Input: part model. Units: mm. Frame: model coordinates. Face numbers are marked on the shaded views. A direction names the side the tool comes from. Coordinates: 2 decimals unless noted, no trailing zeros. Write each loop counter-clockwise with the first axis right and the second up, starting at its lowest first coordinate (ties: lowest second). Pieces come first, ordered by that corner, then holes.
1) Draft query along Z for the marked faces 1, 2 and 3. Return one class per face: pulls with the +Z half, pulls with the -Z half, needs draft (parallel to the pull), parting line crosses it, or undercut.
2) Section query B-B (y = 0). Output: boundary loops of the cut face in (x, z), then the cut area to 3 significant figures.
3) Set-up query: the marked faces 4 and 5. Return all of +Z, -Z, +X, -X, +Y, -Y with unobstructed straight access to the full face (end or side cutting, diameter ignored); none if empty.
4) Pin query (flat end, axial travel): pin 1 Ø1 at (y, z) = (-18, 0.5) entering from +X; pin 2 Ø10 at (x, z) = (4.5, 4.5) entering from +Y; pin 3 Ø7 at (x, y) = (0, 0) entering from +Z; pin 4 Ø2 at (x, z) = (-9, -4) entering from +Y. Return the tip coordinate at first contact, or that it passes through.
5) Section query A-A (z = 0). Output: boundary loops of the cut face in (x, y).
6) Section query D-D (x = 0). Output: boundary loops of the cut face in (y, z), then the cut area to 3 significant figures.
7) Section query C-C (z = -5.75). Output: boundary loops of the cut face in (x, y), then the cut area to 3 significant figures.
8) Line query: L1, parallel to X at y = -54, z = 0; L2, parallel to Y at x = 0, z = 0.55; L3, parallel to Z at x = 8.5, y = -26.5. Output: solid intervals per line, ascending.
from build123d import *

# Parameters (mm, degrees)
SKETCH4_W           = 18
SKETCH4_H           = 18
BOSS_EXTRUDE2_DEPTH = 9
SKETCH5_R           = 3.15
CUT_EXTRUDE1_DEPTH  = 18
SKETCH6_R           = 6
CUT_EXTRUDE2_DEPTH  = 7.25
CUT_EXTRUDE2_DRAFT  = -2
SKETCH8_R           = 6
CUT_EXTRUDE3_DEPTH  = 7.25
CUT_EXTRUDE3_DRAFT  = -2
CHAMFER1_SIZE       = 5
SKETCH13_W          = 18
SKETCH13_H          = 18
BOSS_EXTRUDE4_DEPTH = 50.25
SKETCH14_W          = 35
SKETCH14_H          = 18.08381725
BOSS_EXTRUDE5_DEPTH = 8
SKETCH15_R          = 3.4
CUT_EXTRUDE4_DEPTH  = 8
SKETCH16_R          = 3.4
CUT_EXTRUDE5_DEPTH  = 8


with BuildPart() as part:
    # Sketch4 → Boss-Extrude2 (new, symmetric)
    with BuildSketch(Plane(origin=(0, 0, 0), x_dir=(1, 0, 0), z_dir=(0, 1, 0))):
        Rectangle(SKETCH4_W, SKETCH4_H)
    extrude(amount=BOSS_EXTRUDE2_DEPTH, both=True)

    # Sketch5 → Cut-Extrude1 (cut)
    with BuildSketch(Plane.XY.offset(9)):
        Circle(SKETCH5_R)
    extrude(amount=-CUT_EXTRUDE1_DEPTH, mode=Mode.SUBTRACT)


with BuildPart() as cut_extrude2_tool:
    # Sketch6 → Cut-Extrude2 (with draft: the straight prism first)
    with BuildSketch(Plane.XY.offset(9)):
        Circle(SKETCH6_R)
    extrude(amount=-CUT_EXTRUDE2_DEPTH)
    # Cut-Extrude2: the draft: its side faces are tilted about the plane it starts from
    cut_extrude2_sides = [cut_extrude2_tool.faces().sort_by_distance(p)[0] for p in [
        (-6, 0, 5.375),
    ]]
    draft(cut_extrude2_sides, Plane.XY.offset(9), CUT_EXTRUDE2_DRAFT)


with BuildPart() as part_1:
    add(part.part)

    # Cut-Extrude2: cut by cut_extrude2_tool
    add(cut_extrude2_tool.part, mode=Mode.SUBTRACT)


with BuildPart() as cut_extrude3_tool:
    # Sketch8 → Cut-Extrude3 (with draft: the straight prism first)
    with BuildSketch(Plane(origin=(0, 0, -9), x_dir=(-1, 0, 0), z_dir=(0, 0, -1))):
        Circle(SKETCH8_R)
    extrude(amount=-CUT_EXTRUDE3_DEPTH)
    # Cut-Extrude3: the draft: its side faces are tilted about the plane it starts from
    cut_extrude3_sides = [cut_extrude3_tool.faces().sort_by_distance(p)[0] for p in [
        (6, 0, -5.375),
    ]]
    draft(cut_extrude3_sides, Plane(origin=(0, 0, -9), x_dir=(-1, 0, 0), z_dir=(0, 0, -1)), CUT_EXTRUDE3_DRAFT)


with BuildPart() as part_2:
    add(part_1.part)

    # Cut-Extrude3: cut by cut_extrude3_tool
    add(cut_extrude3_tool.part, mode=Mode.SUBTRACT)

    # Chamfer1
    # the kernel refuses this chamfer: 5 mm, written as the material it takes off along each edge
    with BuildSketch(Plane(origin=(-9, 9, 21.85841494), x_dir=(-0.027495876610586317, -0.9996219169112968, 0), z_dir=(0, 0, -1)), Plane(origin=(-21.85841494, 9, -9), x_dir=(0, -0.9996219169112968, -0.027495876610586317), z_dir=(1, 0, 0))) as chamfer1_piece_1:
        Polygon((CHAMFER1_SIZE * 0.999621916911, -CHAMFER1_SIZE * 0.0274958766106), (-CHAMFER1_SIZE * 0.0274958766106, -CHAMFER1_SIZE * 0.999621916911), (0, 0), align=None)
    extrude(amount=43.71682988, mode=Mode.SUBTRACT)
    with BuildSketch(Plane(origin=(21.85841494, 9, 9), x_dir=(0, 0.027495876610586317, -0.9996219169112968), z_dir=(-1, 0, 0)), Plane(origin=(9, 9, -21.85841494), x_dir=(-0.9996219169112968, 0.027495876610586317, 0), z_dir=(0, 0, 1))) as chamfer1_piece_2:
        Polygon((CHAMFER1_SIZE * 0.999621916911, CHAMFER1_SIZE * 0.0274958766106), (-CHAMFER1_SIZE * 0.0274958766106, CHAMFER1_SIZE * 0.999621916911), (0, 0), align=None)
    extrude(amount=43.71682988, mode=Mode.SUBTRACT)

    # Sketch13 → Boss-Extrude4 (add)
    with BuildSketch(Plane.XZ.offset(9)):
        Rectangle(SKETCH13_W, SKETCH13_H)
    extrude(amount=BOSS_EXTRUDE4_DEPTH)

    # Sketch14 → Boss-Extrude5 (add)
    with BuildSketch(Plane(origin=(0, -59.25, 0), x_dir=(-1, 0, 0), z_dir=(0, -1, 0))):
        Rectangle(SKETCH14_W, SKETCH14_H)
    extrude(amount=-BOSS_EXTRUDE5_DEPTH)

    # Sketch15 → Cut-Extrude4 (cut)
    with BuildSketch(Plane(origin=(0, -51.25, 0), x_dir=(1, 0, 0), z_dir=(0, 1, 0))):
        with Locations(Location((-13.069976583, 0, 0), (0, 0, 270))):
            Circle(SKETCH15_R)
    extrude(amount=-CUT_EXTRUDE4_DEPTH, mode=Mode.SUBTRACT)

    # Sketch16 → Cut-Extrude5 (cut)
    with BuildSketch(Plane(origin=(0, -51.25, 0), x_dir=(1, 0, 0), z_dir=(0, 1, 0))):
        with Locations(Location((13.194452551, 0, 0), (0, 0, 270))):
            Circle(SKETCH16_R)
    extrude(amount=-CUT_EXTRUDE5_DEPTH, mode=Mode.SUBTRACT)


solid = part_2.part
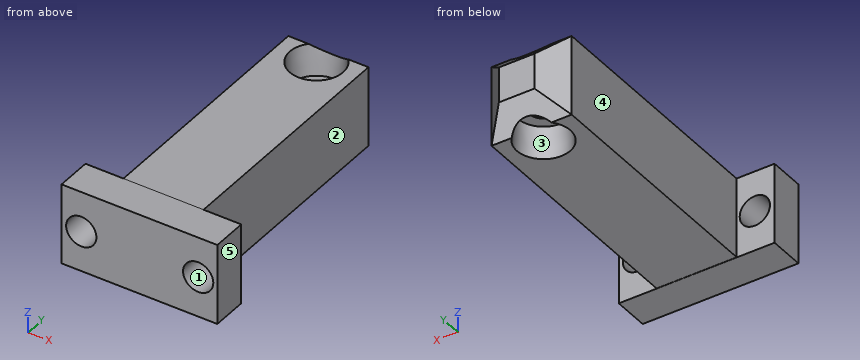
Answer:
1. face 1: undercut
1. face 2: needs draft
1. face 3: pulls with the -Z half
2. outline: (-9, -9) - (-6, -9) - (-5.75, -1.75) - (-3.15, -1.75) - (-3.15, 1.75) - (-5.75, 1.75) - (-6, 9) - (-9, 9) - close; (3.15, -1.75) - (5.75, -1.75) - (6, -9) - (9, -9) - (9, 9) - (6, 9) - (5.75, 1.75) - (3.15, 1.75) - close
2. area: 132 mm2
3. face 4: +Z, -Z, -X, +Y
3. face 5: +Z, -Z, +X, +Y, -Y
4. pin 1: stops at x = 9
4. pin 2: stops at y = 9
4. pin 3: stops at z = 1.75
4. pin 4: stops at y = 5
5. outline: (-17.5, -59.25) - (-16.47, -59.25) - (-16.47, -51.25) - (-17.5, -51.25) - close; (-9.67, -59.25) - (9.79, -59.25) - (9.79, -51.25) - (9, -51.25) - (9, 4) - (4, 9) - (-4, 9) - (-9, 4) - (-9, -51.25) - (-9.67, -51.25) - close; (16.59, -59.25) - (17.5, -59.25) - (17.5, -51.25) - (16.59, -51.25) - close; hole circle Ø6.3 at (0, 0)
6. outline: (-59.25, -9.04) - (-51.25, -9.04) - (-51.25, -9) - (-6, -9) - (-5.75, -1.75) - (-3.15, -1.75) - (-3.15, 1.75) - (-5.75, 1.75) - (-6, 9) - (-51.25, 9) - (-51.25, 9.04) - (-59.25, 9.04) - close; (3.15, -1.75) - (5.75, -1.75) - (5.93, -7.07) - (9, -4) - (9, 4) - (5.93, 7.07) - (5.75, 1.75) - (3.15, 1.75) - close
6. area: 1,020 mm2
7. outline: (-17.5, -59.25) - (17.5, -59.25) - (17.5, -51.25) - (9, -51.25) - (9, 4) - (5.75, 7.25) - (-5.75, 7.25) - (-9, 4) - (-9, -51.25) - (-17.5, -51.25) - close; hole circle Ø11.77 at (0, 0)
7. area: 1,210 mm2
8. L1: x = -17.5 to -16.47, -9.67 to 9.79, 16.59 to 17.5
8. L2: y = -59.25 to -3.15, 3.15 to 9
8. L3: z = -9 to 9
